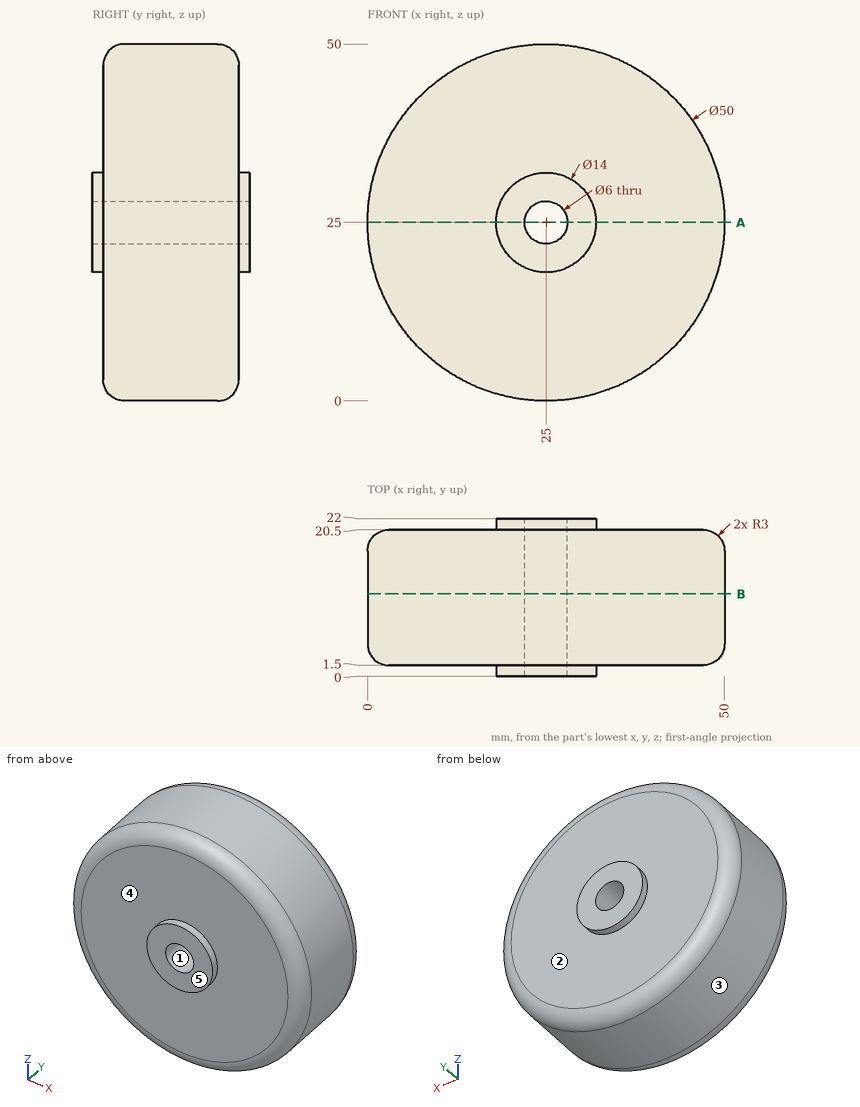
The drawing under review shows one solid part. Ordinate dimensions are in mm from its lowest x, y, z. A direction names the side the tool comes from. Give positions to 0.01 mm unless a question says otherwise; leave off trailing zeros. Loops run counter-clockwise (first coordinate to the right, second up) from the corner with the lowest first, then second, coordinate; pieces in that order, holes last. Notation, with made-up numbers: M 47,33 L 71,33 A14 cw 71,57 Z; hole C -3,-38.75 d7. An arc over 180 degrees is marked long. One line per question, with ' | ' between items. Start each with the question number.
1. To check wall thickness, follow L1, parallel to X at y = 12.75, z = 25; L2, parallel to Y at x = 11, z = 23. State the ranges of each line that lie inside material, in increasing order.
2. Add section B-B (y = 11.5). Write out the cut boundary in (x, z), plus the area to 3 significant figures.
3. Insertion check: P1, Ø8, axis at x = 43, y = 6, coming from the +Z side; P2, Ø5, axis at x = 34, y = 14.5, coming from the -Z side; P3, Ø5.5, axis at x = 25, z = 25, coming from the -Y side; P4, Ø6, axis at x = 13, z = 8.5, coming from the +Y side. Each pin has a flat end and moves straight along its axis. Give the tip position at first contact, or say it passes through.
4. For the marked faces 4 and 5, list the 3-axis set-ups (+Z, -Z, +X, -X, +Y, -Y) from which the entire face can be reached by the end or side of a thin tool; tool diameter is ignored.
5. Add section A-A (z = 25). Write out the cut boundary in (x, y).
6. The part is to be moulded in two halves that separate along X. For the marked faces 1, 2 and 3, say which applies: released by +X, released by -X, zero draft, split by the parting line, or undercut.
Worked out:
1) L1: x = 0 to 22, 28 to 50 | L2: y = 1.5 to 20.5
2) outline: C 25,25 d50; hole C 25,25 d6 | area: 1,940 mm²
3) P1: stops at z = 45.71 | P2: stops at z = 0.86 | P3: passes through | P4: stops at y = 20.5
4) face 4: -Y | face 5: +Z, -Z, +X, -X, -Y
5) outline: M 0,4.5 A3 ccw 3,1.5 L 18,1.5 L 18,0 L 22,0 L 22,22 L 18,22 L 18,20.5 L 3,20.5 A3 ccw 0,17.5 Z; M 28,0 L 32,0 L 32,1.5 L 47,1.5 A3 ccw 50,4.5 L 50,17.5 A3 ccw 47,20.5 L 32,20.5 L 32,22 L 28,22 Z
6) face 1: undercut | face 2: zero draft | face 3: split by the parting line
